from build123d import *

# Parameters (mm, degrees)
CROQUIS1_R              = 20
SALIENTE_EXTRUIR1_DEPTH = 50
CROQUIS2_R              = 20
SALIENTE_EXTRUIR2_DEPTH = 50


with BuildPart() as part:
    # Croquis1 → Saliente-Extruir1 (new body)
    with BuildSketch(Plane.XY):
        with BuildLine():
            Line((140, -145), (200, -145))
            ThreePointArc((200, -145), (0, 30), (-200, -145))
            ThreePointArc((-200, -145), (-170, -175), (-140, -145))
            ThreePointArc((-140, -145), (0, -30), (140, -145))
        make_face()
        Circle(CROQUIS1_R, mode=Mode.SUBTRACT)
        with Locations((-170, -145)):
            Circle(CROQUIS1_R, mode=Mode.SUBTRACT)
    extrude(amount=SALIENTE_EXTRUIR1_DEPTH)

    # Croquis2 → Saliente-Extruir2 (add)
    with BuildSketch(Plane.XZ.offset(145)):
        with Locations((170, 25)):
            Circle(CROQUIS2_R)
    extrude(amount=SALIENTE_EXTRUIR2_DEPTH)


solid = part.part
Could you check a few things on this model? Use its own coordinates, in mm. Round coordinates to 2 decimals unless told otherwise and drop trailing zeros. Order: outer loops, then holes, each group sorted by start corner. A loop starts at its lowest first (then second) coordinate and runs counter-clockwise, first axis right, second up. Notation, with made-up numbers: M 18,69 L 49,69 A29 ccw 49,90 Z; hole C -14.5,69.25 d9. An arc over 180 degrees is marked long. One line per item, written item: value.
(1) Imagine slicing it at C-C (z = 25). Write out the boundary of the cut face in (x, y), and give its area (3 significant figures).
Ans:
outline: M -200,-145 A30 ccw -140,-145 A142.72 cw 140,-145 L 150,-145 L 150,-195 L 190,-195 L 190,-145 L 200,-145 A201.79 ccw Z; hole C -170,-145 d40; hole C 0,0 d40
area: 29,900 mm^2
(2) I'm going to push flat-ended pins straight in: P1, Ø24, axis at x = -170, y = -145, coming from the -Z side; P2, Ø10, axis at y = -53.5, z = 12.5, coming from the +X side; P3, Ø5, axis at y = -24, z = 17.5, coming from the +X side; P4, Ø1, axis at y = -98.5, z = 7.5, coming from the -X side. Where does each tip first touch, or does it pass through?
Ans:
P1: passes through
P2: stops at x = 166.98
P3: stops at x = 140.03
P4: stops at x = -188.2
(3) Imagine slicing it at A-A (x = 0). Write out the boundary of the cut face in (y, z).
Ans:
outline: M -30,0 L -20,0 L -20,50 L -30,50 Z; M 20,0 L 30,0 L 30,50 L 20,50 Z
(4) Imagine slicing it at B-B (y = 0). Write out the boundary of the cut face in (x, z).
Ans:
outline: M -105.86,0 L -20,0 L -20,50 L -105.86,50 Z; M 20,0 L 105.86,0 L 105.86,50 L 20,50 Z
(5) I need wall thicknesses on line 1 along X through (y, z) = (-129, 29); line 2 along X through (y, z) = (-104, 37); line 3 along X through (y, z) = (-59, 39.5). Which ranges of each line are inside material? Lowest first, please. Write a range as from..to.
Ans:
line 1: x = -197.2..-182, -158..-135.86, 135.86..197.2
line 2: x = -190.06..-125.08, 125.08..190.06
line 3: x = -167.32..-86.24, 86.24..167.32
(6) Imagine slicing it at D-D (y = -137.5). Write out the boundary of the cut face in (x, z), and give its area (3 significant figures).
Ans:
outline: M -198.85,0 L -188.54,0 L -188.54,50 L -198.85,50 Z; M -151.46,0 L -138.3,0 L -138.3,50 L -151.46,50 Z; M 138.3,0 L 198.85,0 L 198.85,50 L 138.3,50 Z
area: 4,200 mm^2
(7) If we mould it in two halves opening along Y, with no side actions, what happens to faces 1 (the cylindrical face through (-189.98, -144.12, 24.65)), 2 (the cylindrical face through (150.02, -169.65, 25.88)), 3 (the cylindrical face through (4.06, 29.96, 24.65)), 4 (the flat face through (149.6, -145, 24.6))? For each: released by +Y, released by -Y, zero draft, split by the parting line, or undercut.
Ans:
face 1: undercut
face 2: zero draft
face 3: released by +Y
face 4: released by -Y
